```python
from build123d import *

# Parameters (mm, degrees)
F0_W     = 75
F0_H     = 100
F1_DEPTH = 12.5
F2_R     = 7.5
F3_DEPTH = 50


with BuildPart() as f1:
    # F0 (on Front) → F1 (new body, symmetric)
    with BuildSketch(Plane.XZ):
        Rectangle(F0_W, F0_H)
    extrude(amount=F1_DEPTH, both=True)

    # F2 (on Right) → F3 (join, symmetric)
    with BuildSketch(Plane.YZ):
        with Locations((0, 37.5)):
            Circle(F2_R)
    extrude(amount=F3_DEPTH, both=True)


solid = f1.part
```
The model under review builds one solid part; all positions refer to its coordinate system, in mm. A direction names the side the tool comes from. Coordinates: 2 decimals unless noted, no trailing zeros. Order: outer loops, then holes, each group sorted by start corner. A loop starts at its lowest first (then second) coordinate and runs counter-clockwise, first axis right, second up. Notation, with made-up numbers: (78, -15.75) -> (83, -15.75) arc R29 cw to (83, 14.25) -> close; hole circle Ø11 at (12, -13.5). An arc over 180 degrees is marked (long way). Answer in a Markdown table with one row per item. Add a question column.
Item 1: We need section C-C on x = 44.5. Write out the cut boundary in (y, z).
Item 2: Clearance check with flat-ended pins moving along their axes: pin 1 (2 mm diameter, centred on y = 8.5, z = 12.5, fed in from +X); pin 2 (5 mm diameter, centred on y = -6, z = -37, fed in from -X). State where each tip first meets the part, or that it passes through.
Item 3: Machinability: for faces 1 (the flat face through (-1, -12.5, 1)), 2 (the cylindrical face through (43.84, -1.63, 30.18)), 3 (the cylindrical face through (-43.66, -1.63, 30.18)), which of the approach directions +Z, -Z, +X, -X, +Y, -Y give a long, thin tool a straight path to every point of the face, cutting with its end or side? Answer none if there is none.
Item 4: To check wall thickness, follow probe 1 along X at (y, z) = (-3.5, 2); probe 2 along Z at (x, y) = (-42.5, -5). State the ranges of each line that lie inside material, in increasing order.
Item 5: We need section D-D on z = -29. Write out the cut boundary in (x, y), plus the area to 4 significant figures.
Item 6: We need section A-A on z = 37.5. Write out the cut boundary in (x, y).
Item 7: We need section B-B on y = 0. Write out the cut boundary in (x, z), plus the area to 4 significant figures.
Final values:
| question | item | result |
|---|---|---|
| 1 | outline | circle Ø15 at (0, 37.5) |
| 2 | pin 1 | stops at x = 37.5 |
| 2 | pin 2 | stops at x = -37.5 |
| 3 | face 1 | +Z, -Z, +X, -X, -Y |
| 3 | face 2 | +X |
| 3 | face 3 | -X |
| 4 | probe 1 | x = -37.5 to 37.5 |
| 4 | probe 2 | z = 31.91 to 43.09 |
| 5 | outline | (-37.5, -12.5) -> (37.5, -12.5) -> (37.5, 12.5) -> (-37.5, 12.5) -> close |
| 5 | area | 1,875 mm2 |
| 6 | outline | (-50, -7.5) -> (-37.5, -7.5) -> (-37.5, -12.5) -> (37.5, -12.5) -> (37.5, -7.5) -> (50, -7.5) -> (50, 7.5) -> (37.5, 7.5) -> (37.5, 12.5) -> (-37.5, 12.5) -> (-37.5, 7.5) -> (-50, 7.5) -> close |
| 7 | outline | (-50, 30) -> (-37.5, 30) -> (-37.5, -50) -> (37.5, -50) -> (37.5, 30) -> (50, 30) -> (50, 45) -> (37.5, 45) -> (37.5, 50) -> (-37.5, 50) -> (-37.5, 45) -> (-50, 45) -> close |
| 7 | area | 7,875 mm2 |
